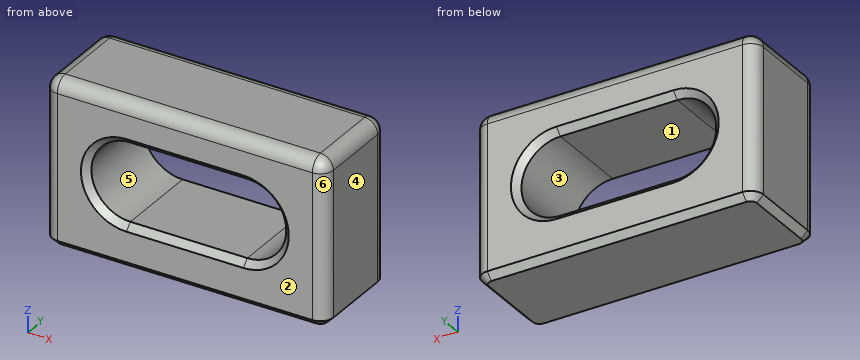
```python
from build123d import *

# Parameters (mm, degrees)
SKETCH004_W     = 21.638793
SKETCH004_H     = 12.638793
PAD003_DEPTH    = 7.5
FILLET002_R     = 1
CHAMFER003_SIZE = 0.5
CHAMFER004_SIZE = 0.5


with BuildPart() as part:
    # Sketch004 → Pad003 (new body)
    with BuildSketch(Plane.XZ):
        with Locations((-10.819396, 6.319396)):
            Rectangle(SKETCH004_W, SKETCH004_H)
        with BuildLine():
            ThreePointArc((-6.319396, 3.319396), (-3.319396, 6.319396), (-6.319396, 9.319396))
            Line((-6.319396, 9.319396), (-15.319396, 9.319396))
            ThreePointArc((-15.319396, 9.319396), (-18.319396, 6.319396), (-15.319396, 3.319396))
            Line((-6.319396, 3.319396), (-15.319396, 3.319396))
        make_face(mode=Mode.SUBTRACT)
    extrude(amount=PAD003_DEPTH)

    # Fillet002
    fillet002_edges = [part.edges().sort_by_distance(p)[0] for p in [
        (-21.638793, 0, 6.319396),
        (-10.819396, 0, 12.638793),
        (-10.819396, -7.5, 12.638793),
        (-21.638793, -3.75, 12.638793),
        (-21.638793, -7.5, 6.319396),
        (0, 0, 6.319396),
        (0, -3.75, 12.638793),
        (0, -7.5, 6.319396),
    ]]
    fillet(fillet002_edges, radius=FILLET002_R)

    # Chamfer003
    chamfer003_edges = [part.edges().sort_by_distance(p)[0] for p in [
        (-10.819396, 0, 0),
    ]]
    chamfer(chamfer003_edges, length=CHAMFER003_SIZE)

    # Chamfer004
    chamfer004_edges = [part.edges().sort_by_distance(p)[0] for p in [
        (-10.819396, 0, 3.319396),
        (-10.819396, -7.5, 3.319396),
    ]]
    chamfer(chamfer004_edges, length=CHAMFER004_SIZE)


with BuildPart() as part_1:
    # Body004 placement: moved
    add(part.part.moved(Location((25.42, 22.43, -4.7))))


solid = part_1.part
```
Source: CAD feature listing. Evaluate the final solid. Frame: model axes, mm. Face numbers are marked on the shaded views. A direction names the side the tool comes from. Round coordinates to 2 decimals unless told otherwise and drop trailing zeros. Loops run counter-clockwise (first coordinate to the right, second up) from the corner with the lowest first, then second, coordinate; pieces in that order, holes last.
(1) Pull-direction query (X, two-part tool) for the marked faces 1, 2, 3 and 4; classes: +X half, -X half, draft (parallel to the pull), parting line (faces both ways), or undercut.
From the geometry:
face 1: undercut
face 2: draft
face 3: undercut
face 4: +X half
(2) Section query B-B (y = 21). Output: boundary loops of the cut face in (x, z), and give its area (3 significant figures).
From the geometry:
outline: (3.78, -4.2) - (4.28, -4.7) - (24.92, -4.7) - (25.42, -4.2) - (25.42, 6.94) arc R1 ccw to (24.42, 7.94) - (4.78, 7.94) arc R1 ccw to (3.78, 6.94) - close; hole (10.1, -1.38) - (19.1, -1.38) arc R3 ccw to (19.1, 4.62) - (10.1, 4.62) arc R3 ccw to start
area: 191 mm2
(3) Section query A-A (x = 12.5). Output: boundary loops of the cut face in (y, z).
From the geometry:
outline: (14.93, -4.2) - (15.43, -4.7) - (21.93, -4.7) - (22.43, -4.2) - (22.43, -1.88) - (21.93, -1.38) - (15.43, -1.38) - (14.93, -1.88) - close; (14.93, 5.12) - (15.43, 4.62) - (21.93, 4.62) - (22.43, 5.12) - (22.43, 6.94) arc R1 ccw to (21.43, 7.94) - (15.93, 7.94) arc R1 ccw to (14.93, 6.94) - close
(4) Material intervals for probe 1 along Z at (x, y) = (12.75, 19.25); probe 2 along X at (y, z) = (17.75, 1.5); probe 3 along Z at (x, y) = (7.75, 20), sorted ascending.
From the geometry:
probe 1: z = -4.7 to -1.38, 4.62 to 7.94
probe 2: x = 3.78 to 7.1, 22.1 to 25.42
probe 3: z = -4.7 to -0.24, 3.48 to 7.94
(5) Access query for the marked faces 5 and 6. Directions: +Z, -Z, +X, -X, +Y, -Y. A direction counts if a zero-diameter tool reaches every point of the face in a straight line with its end or side. Return the directions, or none.
From the geometry:
face 5: +Y, -Y
face 6: +Z, -Z, +X, -Y
